from build123d import *

# Parameters (mm, degrees)
F0_W     = 104.8938632011
F0_H     = 127.0728558302
F1_DEPTH = 68.58
F1_TAPER = 3
F2_R     = 5.08
F3_T     = -2.54


with BuildPart() as f1:
    # F0 (on Top) → F1 (new body)
    with BuildSketch(Plane.XY):
        with Locations((52.4469316006, 63.5364279151)):
            Rectangle(F0_W, F0_H)
    extrude(amount=F1_DEPTH, taper=F1_TAPER)

    # F2
    f2_edges = [f1.edges().sort_by_distance(p)[0] for p in [
        (103.0968, 1.797063, 34.29),
        (103.0968, 125.275793, 34.29),
        (1.797063, 125.275793, 34.29),
        (1.797063, 1.797063, 34.29),
        (3.594126, 63.536428, 68.58),
        (52.446932, 3.594126, 68.58),
        (101.299738, 63.536428, 68.58),
        (52.446932, 123.47873, 68.58),
    ]]
    fillet(f2_edges, radius=F2_R)

    # F3
    f3_openings = [f1.faces().sort_by_distance(p)[0] for p in [
        (52.446932, 63.536428, 0),
    ]]
    offset(amount=F3_T, openings=f3_openings)


solid = f1.part
Input: part model. Units: mm. Frame: model coordinates. A direction names the side the tool comes from. Coordinates: 2 decimals unless noted, no trailing zeros. Order: outer loops, then holes, each group sorted by start corner. A loop starts at its lowest first (then second) coordinate and runs counter-clockwise, first axis right, second up. Notation, with made-up numbers: M -1,-8.5 L 30,-8.5 A13 cw 30,4.5 Z; hole C -18.5,85.25 d9. An arc over 180 degrees is marked long. One line per question, with ' | ' between items.
Item 1: Pin query (flat end, axial travel): pin 1 (5 mm diameter, centred on y = 98.5, z = 53, fed in from -X); pin 2 (10 mm diameter, centred on x = 45, y = 59, fed in from -Z); pin 3 (12 mm diameter, centred on y = 78, z = 27, fed in from -X). Return the tip coordinate at first contact, or that it passes through.
Geometry results:
pin 1: stops at x = 2.65 | pin 2: stops at z = 66.04 | pin 3: stops at x = 1.1
Item 2: Reachability of faces 1 (the flat face through (53.11, 1.648, 31.437)), 2 (the cylindrical face through (99.9, 122.11, 32.29)) from +Z, -Z, +X, -X, +Y, -Y: full face, straight path, thin tool, end or side. Return the list, or none.
Geometry results:
face 1: +Z, +X, -X, -Y | face 2: -Z
Item 3: Section B-B (y = 13). Output: boundary loops of the cut face in (x, z).
Geometry results:
outline: M 0,0 L 2.54,0 L 5.88,63.63 A2.54 cw 8.41,66.04 L 96.48,66.04 A2.54 cw 99.02,63.63 L 102.35,0 L 104.89,0 L 101.55,63.77 A5.08 ccw 96.48,68.58 L 8.41,68.58 A5.08 ccw 3.34,63.77 Z
Item 4: Section A-A (x = 12). Output: boundary loops of the cut face in (y, z).
Geometry results:
outline: M 0,0 L 2.54,0 L 5.88,63.63 A2.54 cw 8.41,66.04 L 118.66,66.04 A2.54 cw 121.19,63.63 L 124.53,0 L 127.07,0 L 123.73,63.77 A5.08 ccw 118.66,68.58 L 8.41,68.58 A5.08 ccw 3.34,63.77 Z
Item 5: Draft query along Y for faces 3 (the flat face through (52, 64, 68.58)), 4 (the flat face through (100.706, 64.355, 31.371)), 5 (the cylindrical face through (3.14, 3.22, 32.36)), 6 (the cylindrical face through (4.958, 122.075, 32.285)). Return one class per face: released by +Y, released by -Y, zero draft, split by the parting line, or undercut.
Geometry results:
face 3: zero draft | face 4: undercut | face 5: released by -Y | face 6: undercut
Item 6: Ray query, line 1 along Z through (x, y) = (89, 54); line 2 along Y through (x, z) = (36.5, 36); line 3 along Y through (x, z) = (40.5, 7). Return the intervals inside material, ascending.
Geometry results:
line 1: z = 66.04 to 68.58 | line 2: y = 1.89 to 4.43, 122.64 to 125.19 | line 3: y = 0.37 to 2.91, 124.16 to 126.71
